Autodesk Inventor part; units mm, degrees
ref_plane "YZ Plane" through (0, 0, 0) normal (1, 0, 0) x (0, 1, 0)
ref_plane "XZ Plane" through (0, 0, 0) normal (0, 1, 0) x (-1, 0, 0)
ref_plane "XY Plane" through (0, 0, 0) normal (0, 0, 1) x (1, 0, 0)
ref_plane "Work Plane2" through (-2.3036, 0, -9.6783) normal (1, 0, 0) x (0, 0, -1)
sketch "Sketch1" plane through (-2.3036, 0, -9.6783) normal (1, 0, 0) x (0, 0, -1)
  line L0 (0, 0) -> (-5.2832, 0)
  line L1 (-2.6416, 0) -> (-2.6416, 10.3378)
  line L2 (-2.6416, 10.3378) -> (-2.6416, 11.1315)
  line L3 (-2.6416, 0) -> (-2.6416, 11.5316)
  point P0 (-9.6783, 0)
  dimension "d24" = 11.5316
ref_plane "Work Plane1" through (-2.3036, 0, -9.6783) normal (1, 0, 0) x (0, 0, -1)
sketch "Sketch2" plane through (-2.3036, 0, -9.6783) normal (1, 0, 0) x (0, 0, -1)
  point P0 (-9.6783, 0)
ref_plane "Work Plane3" through (-2.3036, 0, -9.6783) normal (1, 0, 0) x (0, 0, -1)
ref_plane "Work Plane6" through (-7.5868, 0, -9.6783) normal (-1, 0, 0) x (0, 0, 1)
sketch "Sketch5" plane through (-7.5868, 0, -9.6783) normal (-1, 0, 0) x (0, 0, 1)
  line L0 (0, 0) -> (5.2832, 0)
  line L1 (2.6416, 0) -> (2.6416, 14.7688)
  line L2 (2.6416, 14.7688) -> (2.6416, 15.7975)
  line L3 (2.6416, 15.7975) -> (2.6416, 18.2867)
  circle A0 centre (2.6416, 15.7975) radius 1.524
  point P0 (9.6783, 0)
  dimension "d25" = 1.0287
  dimension "d26" = 2.4892
  dimension "d27" = 3.048
ref_plane "Work Plane5" through (-7.5868, 0, -9.6783) normal (0, -1, 0) x (1, 0, 0)
sketch "Sketch6" plane through (-7.5868, 0, -9.6783) normal (0, -1, 0) x (1, 0, 0)
  line L0 (0, 0) -> (0, 5.2832)
  line L1 (5.2832, 0) -> (0, 0)
  line L2 (0, 5.2832) -> (5.2832, 5.2832)
  line L3 (5.2832, 5.2832) -> (5.2832, 0)
  line L4 (5.2832, 0) -> (0, 0)
  line L5 (0, 0) -> (0, 5.2832)
  arc A0 (3.5677, 2.2318) -> (3.582, 3.0171) centre (2.6416, 2.6416) ccw
  circle A1 centre (2.6416, 2.6416) radius 1.4224
  point P0 (7.5868, 9.6783)
  dimension "d35" = 2.8448
extrude "Extrusion3" add sketch "Sketch6" against normal blind 18.288 contours L0 L2 L3 L1 | A1
hole "Hole4" at (-7.5868, 15.7975, -7.0367) direction (1, 0, 0) diameter 3.048 end through all
extrude "Extrusion4" cut sketch "Sketch6" against normal blind 11.684 contours A1
thread "Thread1"
properties part number "rod1"
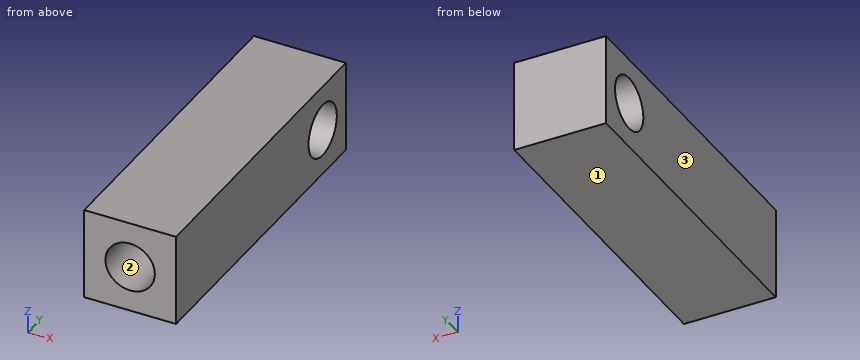
Geometry check sheet. Reference: the model listing, model coordinates, mm. Face numbers are marked on the shaded views. Give positions to 0.01 mm unless a question says otherwise; leave off trailing zeros. Loops run counter-clockwise (first coordinate to the right, second up) from the corner with the lowest first, then second, coordinate; pieces in that order, holes last.
(1) Release check for a two-part mould opening along Z. For the marked faces 1, 2 and 3 record: released by +Z, released by -Z, zero draft, split by the parting line, or undercut.
From the geometry:
face 1: released by -Z
face 2: undercut
face 3: zero draft
(2) Section check C-C on x = -5.6. Record the cut outline in (y, z).
From the geometry:
outline: (0, -9.68) - (18.29, -9.68) - (18.29, -4.4) - (0, -4.4) - (0, -5.77) - (11.68, -5.77) - (11.68, -8.3) - (0, -8.3) - close; hole circle Ø3.05 at (15.8, -7.04)
(3) Depth check by flat-ended pin: pin 1 Ø2.5 at (y, z) = (15.8, -7.04) entering from +X. Enter the tip coordinate at first touch or a pass-through.
From the geometry:
pin 1: passes through
(4) Section check D-D on y = 15. Record the cut outline in (x, z), then the cut area to 3 significant figures.
From the geometry:
outline: (-7.59, -9.68) - (-2.3, -9.68) - (-2.3, -8.34) - (-7.59, -8.34) - close; (-7.59, -5.74) - (-2.3, -5.74) - (-2.3, -4.4) - (-7.59, -4.4) - close
area: 14.2 mm2
(5) Section check A-A on z = -5.85. Record the cut outline in (x, y).
From the geometry:
outline: (-7.59, 0) - (-5.73, 0) - (-5.73, 11.68) - (-4.16, 11.68) - (-4.16, 0) - (-2.3, 0) - (-2.3, 14.84) - (-7.59, 14.84) - close; (-7.59, 16.75) - (-2.3, 16.75) - (-2.3, 18.29) - (-7.59, 18.29) - close
(6) Section check B-B on y = 2.5. Record the cut outline in (x, z).
From the geometry:
outline: (-7.59, -9.68) - (-2.3, -9.68) - (-2.3, -4.4) - (-7.59, -4.4) - close; hole circle Ø2.84 at (-4.95, -7.04)
(7) Thickness scan on L1, parallel to Y at x = -5.6, z = -7.1; L2, parallel to Z at x = -3.85, y = 15.25; L3, parallel to X at y = 3.5, z = -7.1. Record the ranges inside material, lowest first.
From the geometry:
L1: y = 11.68 to 14.27, 17.32 to 18.29
L2: z = -9.68 to -8.46, -5.61 to -4.4
L3: x = -7.59 to -6.37, -3.52 to -2.3
